The model under review builds one solid part; all positions refer to its coordinate system, in mm. A direction names the side the tool comes from. Give positions to 0.01 mm unless a question says otherwise; leave off trailing zeros. Loops run counter-clockwise (first coordinate to the right, second up) from the corner with the lowest first, then second, coordinate; pieces in that order, holes last. Notation, with made-up numbers: M 44.5,9 L 81.5,9 A13 ccw 81.5,18 Z; hole C -29.5,45.25 d8. An arc over 180 degrees is marked long. One line per item, written item: value. Start each with the question number.
Q1. Mouldability with a two-part tool opening along Z and no side actions: class faces 1 (the face through (-5.207, 2.003, -5.092)), 2 (the face through (11.5, 1, 0)), 3 (the face through (10, 2, -4)) as released by +Z, released by -Z, zero draft, split by the parting line, or undercut.
Q2. For faces 4 (the face through (0, 1.5, 0)), 5 (the face through (10, 2, -3.5)), 6 (the face through (0, 0, 0)), 7 (the face through (8.3, 2, 0)), 8 (the face through (10, 2, 4)), list the 3-axis set-ups (+Z, -Z, +X, -X, +Y, -Y) from which the entire face can be reached by the end or side of a thin tool; tool diameter is ignored.
Q3. We need section A-A on y = 1.95. Give the number of separate pieces and of enclosed holes in the cut face, plus the area to 3 significant figures.
Q4. For pin 1 (0.5 mm diameter, centred on x = -8, z = 5, fed in from +Y); pin 2 (1.4 mm diameter, centred on x = 10.5, y = 2.5, fed in from +Z); pin 3 (2 mm diameter, centred on x = -5.5, z = -1.5, fed in from +Y); pin 4 (4 mm diameter, centred on x = -5, z = -2, fed in from -Y), all flat-tipped, find the tip position at first contact; note any pin that passes through.
Q5. We need section B-B on x = -3. Write out the cut boundary in (y, z).
Q6. We need section C-C on z = 0. Write out the cut boundary in (x, y), plus the area to 3 significant figures.
Q7. We need section D-D on x = -6.75. Write out the cut boundary in (y, z).
Q8. To check wall thickness, follow line 1 along Y through (x, z) = (-3.75, -0.75); line 2 along X through (y, z) = (2.2, 3); line 3 along X through (y, z) = (2.15, -3.75). State the ranges of each line that lie inside material, in increasing order. Write a range as from..to.
```python
from build123d import *

# Parameters (mm, degrees)
SKETCH1_W               = 23
SKETCH1_H               = 12
BOSS_EXTRUDE1_DEPTH     = 1.5
SKETCH2_W               = 3.2
SKETCH2_H               = 8
BOSS_EXTRUDE2_DEPTH     = 2
SKETCH3_W               = 7
SKETCH3_H               = 1.3
CUT_EXTRUDE1_DEPTH      = 2.7
SKETCH4_R               = 0.5
BOSS_EXTRUDE3_DEPTH     = 0.69
BOSS_EXTRUDE3_TAPER     = 21
LPATTERN1_COUNT         = 6
LPATTERN1_PITCH         = 2.5
MIRROR1_COPY_1_SKETCH_R = 0.5
MIRROR1_COPY_1_DEPTH    = 0.69
MIRROR1_COPY_1_TAPER    = 21
MIRROR1_COPY_2_SKETCH_R = 0.5
MIRROR1_COPY_2_DEPTH    = 0.69
MIRROR1_COPY_2_TAPER    = 21
MIRROR1_COPY_3_SKETCH_R = 0.5
MIRROR1_COPY_3_DEPTH    = 0.69
MIRROR1_COPY_3_TAPER    = 21
MIRROR1_COPY_4_SKETCH_R = 0.5
MIRROR1_COPY_4_DEPTH    = 0.69
MIRROR1_COPY_4_TAPER    = 21
MIRROR1_COPY_5_SKETCH_R = 0.5
MIRROR1_COPY_5_DEPTH    = 0.69
MIRROR1_COPY_5_TAPER    = 21


with BuildPart() as part:
    # Sketch1 → Boss-Extrude1 (new body)
    with BuildSketch(Plane(origin=(0, 0, 0), x_dir=(1, 0, 0), z_dir=(0, 1, 0))):
        Rectangle(SKETCH1_W, SKETCH1_H)
    extrude(amount=BOSS_EXTRUDE1_DEPTH)

    # Sketch2 → Boss-Extrude2 (add)
    with BuildSketch(Plane(origin=(0, 1.5, 0), x_dir=(1, 0, 0), z_dir=(0, 1, 0))):
        with Locations((9.9, 0)):
            Rectangle(SKETCH2_W, SKETCH2_H)
    extrude(amount=BOSS_EXTRUDE2_DEPTH)

    # Sketch3 → Cut-Extrude1 (cut)
    with BuildSketch(Plane(origin=(11.5, 0, 0), x_dir=(0, 0, -1), z_dir=(1, 0, 0))):
        with Locations((0, 2.35)):
            Rectangle(SKETCH3_W, SKETCH3_H)
    extrude(amount=-CUT_EXTRUDE1_DEPTH, mode=Mode.SUBTRACT)

    # Sketch4 → Boss-Extrude3 (add)
    with BuildSketch(Plane(origin=(0, 1.5, 0), x_dir=(1, 0, 0), z_dir=(0, 1, 0))):
        with Locations((-10.5, 5)):
            Circle(SKETCH4_R)
    boss_extrude3 = extrude(amount=BOSS_EXTRUDE3_DEPTH, taper=BOSS_EXTRUDE3_TAPER)

    # LPattern1: Boss-Extrude3 ×6
    with Locations(*[(i * LPATTERN1_PITCH, 0, 0) for i in range(1, LPATTERN1_COUNT)]):
        add(boss_extrude3)

    # Mirror1: Boss-Extrude3 across plane
    add(boss_extrude3.mirror(Plane.XY))

    # Mirror1 copy 1 sketch → Mirror1 copy 1 (add)
    with BuildSketch(Plane(origin=(2.5, 1.5, 0), x_dir=(1, 0, 0), z_dir=(0, 1, 0))):
        with Locations((-10.5, -5)):
            Circle(MIRROR1_COPY_1_SKETCH_R)
    extrude(amount=MIRROR1_COPY_1_DEPTH, taper=MIRROR1_COPY_1_TAPER)

    # Mirror1 copy 2 sketch → Mirror1 copy 2 (add)
    with BuildSketch(Plane(origin=(5, 1.5, 0), x_dir=(1, 0, 0), z_dir=(0, 1, 0))):
        with Locations((-10.5, -5)):
            Circle(MIRROR1_COPY_2_SKETCH_R)
    extrude(amount=MIRROR1_COPY_2_DEPTH, taper=MIRROR1_COPY_2_TAPER)

    # Mirror1 copy 3 sketch → Mirror1 copy 3 (add)
    with BuildSketch(Plane(origin=(7.5, 1.5, 0), x_dir=(1, 0, 0), z_dir=(0, 1, 0))):
        with Locations((-10.5, -5)):
            Circle(MIRROR1_COPY_3_SKETCH_R)
    extrude(amount=MIRROR1_COPY_3_DEPTH, taper=MIRROR1_COPY_3_TAPER)

    # Mirror1 copy 4 sketch → Mirror1 copy 4 (add)
    with BuildSketch(Plane(origin=(10, 1.5, 0), x_dir=(1, 0, 0), z_dir=(0, 1, 0))):
        with Locations((-10.5, -5)):
            Circle(MIRROR1_COPY_4_SKETCH_R)
    extrude(amount=MIRROR1_COPY_4_DEPTH, taper=MIRROR1_COPY_4_TAPER)

    # Mirror1 copy 5 sketch → Mirror1 copy 5 (add)
    with BuildSketch(Plane(origin=(12.5, 1.5, 0), x_dir=(1, 0, 0), z_dir=(0, 1, 0))):
        with Locations((-10.5, -5)):
            Circle(MIRROR1_COPY_5_SKETCH_R)
    extrude(amount=MIRROR1_COPY_5_DEPTH, taper=MIRROR1_COPY_5_TAPER)


solid = part.part
```
Solved:
1. face 1: undercut
1. face 2: zero draft
1. face 3: released by -Z
2. face 4: +Y
2. face 5: +X
2. face 6: +Z, -Z, +X, -X, -Y
2. face 7: +Z, -Z, -X, +Y
2. face 8: +Z, +X, -X, +Y
3. separate pieces: 13
3. enclosed holes: 0
3. area: 10.7 mm2
4. pin 1: y = 2.19
4. pin 2: z = 4
4. pin 3: y = 1.5
4. pin 4: y = 0
5. outline: M 0,-6 L 1.5,-6 L 1.5,-5.5 L 2.19,-5.24 L 2.19,-4.76 L 1.5,-4.5 L 1.5,4.5 L 2.19,4.76 L 2.19,5.24 L 1.5,5.5 L 1.5,6 L 0,6 Z
6. outline: M -11.5,0 L 11.5,0 L 11.5,1.7 L 8.8,1.7 L 8.8,3 L 11.5,3 L 11.5,3.5 L 8.3,3.5 L 8.3,1.5 L -11.5,1.5 Z
6. area: 37.4 mm2
7. outline: M 0,-6 L 1.5,-6 L 1.5,6 L 0,6 Z
8. line 1: 0..1.5
8. line 2: 8.3..8.8
8. line 3: 8.3..11.5
